```python
from build123d import *

# Parameters (mm, degrees)
SKETCH1_R                 = 8.5
BOSS_EXTRUDE1_DEPTH       = 46
SKETCH2_R                 = 8
BOSS_EXTRUDE2_DEPTH       = 34
CUT_EXTRUDE1_DEPTH        = 81.898084032
CUT_EXTRUDE1_DEPTH_BACK   = 81.898084032
SKETCH3_W                 = 2.5
SKETCH3_H                 = 25.25
FILLET1_R                 = 1
F_6_0MM_DOWEL_HOLE1_D     = 6
F_6_0MM_DOWEL_HOLE1_DEPTH = 32.197418143
F_6_0MM_DOWEL_HOLE1_TIP   = 1.802581857


with BuildPart() as part:
    # Sketch1 → Boss-Extrude1 (new body)
    with BuildSketch(Plane.XY):
        Circle(SKETCH1_R)
    extrude(amount=BOSS_EXTRUDE1_DEPTH)

    # Sketch2 → Boss-Extrude2 (add)
    with BuildSketch(Plane.XY.offset(46)):
        Circle(SKETCH2_R)
    extrude(amount=BOSS_EXTRUDE2_DEPTH)

    # Sketch3 → Cut-Extrude1 (cut, two sides: drawn at the far end of the back side and taken through both)
    with BuildSketch(Plane(origin=(0, 0, 0), x_dir=(1, 0, 0), z_dir=(0, 1, 0)).offset(-CUT_EXTRUDE1_DEPTH_BACK)):
        with Locations((-6.75, -63.625)):
            Rectangle(SKETCH3_W, SKETCH3_H)
    extrude(amount=CUT_EXTRUDE1_DEPTH + CUT_EXTRUDE1_DEPTH_BACK, mode=Mode.SUBTRACT)

    # Fillet1
    fillet1_edges = [part.edges().sort_by_distance(p)[0] for p in [
        (-5.5, 0, 51),
        (-5.5, 0, 76.25),
    ]]
    fillet(fillet1_edges, radius=FILLET1_R)

    # Chamfer1: read off the stored shape, not the designer's step
    # Chamfer1 outline → Chamfer1 (revolve, cut)
    with BuildSketch(Plane.XZ):
        Polygon((8, 80), (7.47339001, 80), (8, 76), align=None)
    revolve(axis=Axis((0, 0, 0), (0, 0, 1)), mode=Mode.SUBTRACT)

    # Ø6.0mm Dowel Hole1
    with Locations(Plane.XY.offset(80)):
        with Locations((0, 0)):
            Hole(F_6_0MM_DOWEL_HOLE1_D / 2, depth=F_6_0MM_DOWEL_HOLE1_DEPTH)
            with Locations((0, 0, -(F_6_0MM_DOWEL_HOLE1_DEPTH + F_6_0MM_DOWEL_HOLE1_TIP / 2))):  # 118° drill point
                Cone(0, F_6_0MM_DOWEL_HOLE1_D / 2, F_6_0MM_DOWEL_HOLE1_TIP, mode=Mode.SUBTRACT)


solid = part.part
```
Could you check a few things on this model? Use its own coordinates, in mm. A direction names the side the tool comes from. Round coordinates to 2 decimals unless told otherwise and drop trailing zeros. Loops run counter-clockwise (first coordinate to the right, second up) from the corner with the lowest first, then second, coordinate; pieces in that order, holes last. Notation, with made-up numbers: (36, -3) - (51, -3) arc R13 ccw to (51, 16) - close; hole circle Ø7 at (-27, 74.5). An arc over 180 degrees is marked (long way). Use CSV: the item, a comma, the result in double quotes.
Item 1: Will these pins go through, and if not, where does the flat tip stop? pin 1 (1.5 mm diameter, centred on x = 6, z = 31, fed in from +Y); pin 2 (2 mm diameter, centred on y = -1.5, z = 38, fed in from +X); pin 3 (10 mm diameter, centred on y = -6.5, z = 26, fed in from -X).
Here are the results:
pin 1,"stops at y = 6.68"
pin 2,"stops at x = 8.49"
pin 3,"stops at x = -8.37"
Item 2: I need wall thicknesses on L1, parallel to Y at x = 0, z = 64.5; L2, parallel to X at y = 0, z = 70; L3, parallel to Y at x = 6.5, z = 64. Which ranges of each line are inside material? Lowest first, please. Write a range as [from, to].
Here are the results:
L1,"y = [-8, -3], [3, 8]"
L2,"x = [-5.5, -3], [3, 8]"
L3,"y = [-4.66, 4.66]"
Item 3: If we section it at B-B on z = 41.5: List the corners of the cut face in (x, y) for me, then the cut area to 3 significant figures.
Here are the results:
outline,"circle Ø17 at (0, 0)"
area,"227 mm²"
Item 4: For faces 1 (the flat face through (3.2, 0.1, 80)), 2 (the flat face through (-5.5, 0, 64)), which set-ups out of +Z, -Z, +X, -X, +Y, -Y let a thin tool reach every point of the face, with its end or its side?
Here are the results:
face 1,"+Z, +X, -X, +Y, -Y"
face 2,"-X, +Y, -Y"
Item 5: If we mould it in two halves opening along Y, with no side actions, what happens to faces 3 (the cylindrical face through (7.39, -3.06, 60.79)), 4 (the conical face through (-0.113, -0.509, 46.313)), 5 (the cylindrical face through (3, 0, 64)), 6 (the flat face through (0, 0, 0))? For each: pulls with the +Y half, pulls with the -Y half, needs draft (parallel to the pull), parting line crosses it, or undercut.
Here are the results:
face 3,"parting line crosses it"
face 4,"undercut"
face 5,"undercut"
face 6,"needs draft"
Item 6: If we section it at A-A on z = 58: List the corners of the cut face in (x, y) for me.
Here are the results:
outline,"(-5.5, -5.81) arc R8 ccw (long way) to (-5.5, 5.81) - close; hole circle Ø6 at (0, 0)"
